```python
from build123d import *

# Parameters (mm, degrees)
CHAMFER1_SIZE = 0.3


with BuildPart() as part:
    # Sketch1 → Revolve1 (revolve)
    with BuildSketch(Plane(origin=(0, 0, 0), x_dir=(0, 0, -1), z_dir=(1, 0, 0))):
        Polygon((-2.975, 11.945), (-2.425, 11.945), (-0.275, 9.77), (-0.275, 9.375), (0.275, 9.375), (0.275, 9.77), (2.425, 11.945), (2.975, 11.945), (5.115, 9.77), (5.115, 7.987), (0.5, 7.987), (0.5, 6.945), (-0.5, 6.945), (-0.5, 7.987), (-5.115, 7.987), (-5.115, 9.77), align=None)
    revolve(axis=Axis((0, 0, 5.115), (0, 0, -1)))

    # Chamfer1
    chamfer1_edges = [part.edges().sort_by_distance(p)[0] for p in [
        (0, -7.987, -5.115),
        (0, -7.987, 5.115),
    ]]
    chamfer(chamfer1_edges, length=CHAMFER1_SIZE)


solid = part.part
```
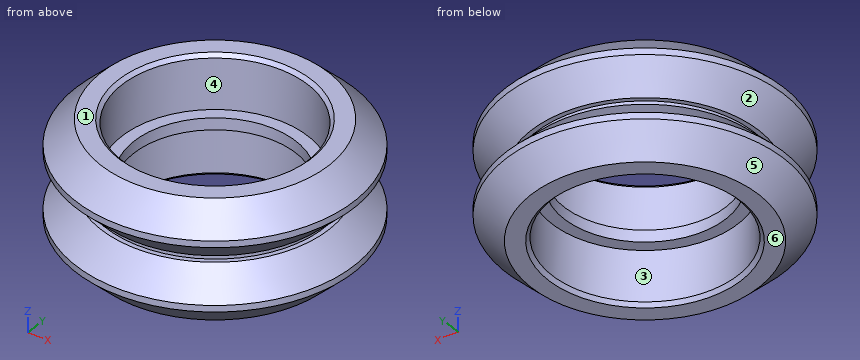
The listing builds one solid part. Answer for the finished solid, in the listing's coordinates (mm). Face numbers are marked on the shaded views. A direction names the side the tool comes from. Round coordinates to 2 decimals unless told otherwise and drop trailing zeros. Answer as CSV lines item,"result". Start each with the question number.
(1) A tool of negligible diameter and unlimited length cuts with its end or side. For the marked faces 1, 2 and 3, from which of +Z, -Z, +X, -X, +Y, -Y can it reach the whole face along a straight path? Write none if from no direction.
(2) Flat-ended cylindrical pins translate along their axes: pin 1 Ø1 at (x, y) = (6.5, 1.5) entering from -Z; pin 2 Ø1 at (y, z) = (9.5, 4) entering from -X; pin 3 Ø4 at (x, z) = (7.5, -0.5) entering from -Y. Find the tip coordinate at first contact, or state that the pin passes through.
(3) Find the intervals of material crossed by probe 1 along X at (y, z) = (0, 2.5) (3 decimals); probe 2 along X at (y, z) = (-2, -1.5); probe 3 along Z at (x, y) = (2, -9.25) (3 decimals), in increasing order. Write a range as from..to.
(4) For a pull along X with two mould halves and no side action, classify the marked faces 4, 5 and 6 as +X half, -X half, draft (parallel to the pull), parting line (faces both ways), or undercut.
Evaluation:
1,face 1,"+Z, +X, -X, +Y, -Y"
1,face 2,"none"
1,face 3,"-Z"
2,pin 1,"z = -0.5"
2,pin 2,"x = -6.58"
2,pin 3,"y = -9.79"
3,probe 1,"-11.945..-7.987, 7.987..11.945"
3,probe 2,"-10.83..-7.73, 7.73..10.83"
3,probe 3,"-5.115..-0.275, 0.275..5.115"
4,face 4,"undercut"
4,face 5,"parting line"
4,face 6,"draft"
